The model under review builds one solid part; all positions refer to its coordinate system, in mm. A direction names the side the tool comes from. Give positions to 0.01 mm unless a question says otherwise; leave off trailing zeros. Loops run counter-clockwise (first coordinate to the right, second up) from the corner with the lowest first, then second, coordinate; pieces in that order, holes last. Notation, with made-up numbers: M 21,80 L 67,80 A10 cw 67,92 Z; hole C -23.5,61 d7. An arc over 180 degrees is marked long. Write item = value, one per line. Start each with the question number.
1. We need section B-B on z = 37. Give the boundary of the cut face in (x, y).
2. For faces 4 (the face through (-12.5, -35, 10)), 5 (the face through (0, 20, 23)), 6 (the face through (-35, 30, 15)), 7 (the face through (0, 40, 16)), 8 (the face through (15, 30, 33)), list the 3-axis set-ups (+Z, -Z, +X, -X, +Y, -Y) from which the entire face can be reached by the end or side of a thin tool; tool diameter is ignored.
3. Draft analysis for pull direction X (two halves, no side actions). For faces 1 (the face through (-15, 30, 33)), 2 (the face through (16, -50, 10)), 3 (the face through (-27.395, -25.35, 10.14)), state which applies: pulls with the +X half, pulls with the -X half, needs draft (parallel to the pull), parting line crosses it, or undercut.
4. We need section D-D on x = -24.5. Give the boundary of the cut face in (y, z), then the cut area to 3 significant figures.
5. For pin 1 (10 mm diameter, centred on y = -31.5, z = 9, fed in from -X); pin 2 (6 mm diameter, centred on y = -6, z = 6.5, fed in from +X); pin 3 (2 mm diameter, centred on x = 27, z = 29, fed in from -Y), all flat-tipped, find the tip position at first contact; note any pin that passes through.
6. We need section A-A on y = 41.5. Give the boundary of the cut face in (x, z).
7. We need section C-C on y = 22. Give the boundary of the cut face in (x, z), then the cut area to 3 significant figures.
8. Wall thickness on line 1 along X through (y, z) = (33, 34); line 2 along Y through (x, z) = (25, 23.5); line 3 along Y through (x, z) = (17.5, 22): over which ranges is each line inside the solid? List them lowest first. Write a range as from..to.
from build123d import *

# Parameters (mm, degrees)
SKETCH_W        = 70
SKETCH_H        = 100
PAD_DEPTH       = 20
POCKET_DEPTH    = 20.001
SKETCH002_W     = 25
SKETCH002_H     = 30
POCKET001_DEPTH = 20.001
SKETCH003_W     = 70
SKETCH003_H     = 30
PAD001_DEPTH    = 20
SKETCH004_W     = 40
SKETCH004_H     = 21.64003
POCKET002_DEPTH = 40.001
SKETCH005_W     = 30
SKETCH005_H     = 38.026675
POCKET003_DEPTH = 15


with BuildPart() as part:
    # Sketch → Pad (new body)
    with BuildSketch(Plane.XY):
        Rectangle(SKETCH_W, SKETCH_H)
    extrude(amount=PAD_DEPTH)

    # Sketch001 → Pocket (cut, through all)
    with BuildSketch(Plane.XY.offset(20)):
        Polygon((35, 0), (35, -50), (20, -50), align=None)
        Polygon((-35, 0), (-35, -50), (-20, -50), align=None)
    extrude(amount=-POCKET_DEPTH, mode=Mode.SUBTRACT)

    # Sketch002 → Pocket001 (cut, through all)
    with BuildSketch(Plane.XY.offset(20)):
        with Locations((0, -35)):
            Rectangle(SKETCH002_W, SKETCH002_H)
    extrude(amount=-POCKET001_DEPTH, mode=Mode.SUBTRACT)

    # Sketch003 → Pad001 (new body)
    with BuildSketch(Plane.XY.offset(20)):
        with Locations((0, 35)):
            Rectangle(SKETCH003_W, SKETCH003_H)
    extrude(amount=PAD001_DEPTH)

    # Sketch004 → Pocket002 (cut, through all)
    with BuildSketch(Plane.XY.offset(40)):
        with Locations((0, 50.820015)):
            Rectangle(SKETCH004_W, SKETCH004_H)
    extrude(amount=-POCKET002_DEPTH, mode=Mode.SUBTRACT)

    # Sketch005 → Pocket003 (cut)
    with BuildSketch(Plane.XY.offset(40)):
        with Locations((0, 31.280009)):
            Rectangle(SKETCH005_W, SKETCH005_H)
    extrude(amount=-POCKET003_DEPTH, mode=Mode.SUBTRACT)


solid = part.part
Final values:
q1.outline = M -35,20 L -15,20 L -15,40 L -20,40 L -20,50 L -35,50 Z; M 15,20 L 35,20 L 35,50 L 20,50 L 20,40 L 15,40 Z
q2.face_4 = +Z, -Z, -Y
q2.face_5 = +Z, +X, -X, -Y
q2.face_6 = +Z, -Z, -X, +Y, -Y
q2.face_7 = +Z, -Z, +Y
q2.face_8 = +Z, +Y, -Y
q3.face_1 = undercut
q3.face_2 = needs draft
q3.face_3 = pulls with the -X half
q4.outline = M -35,0 L 50,0 L 50,40 L 20,40 L 20,20 L -35,20 Z
q4.area = 2,300 mm²
q5.pin_1 = -27.05
q5.pin_2 = 34.1
q5.pin_3 = 20
q6.outline = M -35,0 L -20,0 L -20,40 L -35,40 Z; M 20,0 L 35,0 L 35,40 L 20,40 Z
q7.outline = M -35,0 L 35,0 L 35,40 L 15,40 L 15,25 L -15,25 L -15,40 L -35,40 Z
q7.area = 2,350 mm²
q8.line_1 = -35..-15, 15..35
q8.line_2 = 20..50
q8.line_3 = 20..40
